Read the model definition and answer for the solid it produces. Units are mm, in the model's axes. A direction names the side the tool comes from. Coordinates: 2 decimals unless noted, no trailing zeros. Loops run counter-clockwise (first coordinate to the right, second up) from the corner with the lowest first, then second, coordinate; pieces in that order, holes last.
Autodesk Inventor part; units mm, degrees
ref_plane "YZ Plane" through (0, 0, 0) normal (1, 0, 0) x (0, 1, 0)
ref_plane "XZ Plane" through (0, 0, 0) normal (0, 1, 0) x (-1, 0, 0)
ref_plane "XY Plane" through (0, 0, 0) normal (0, 0, 1) x (1, 0, 0)
sketch "Sketch1" plane through (0, 0, 0) normal (0, 1, 0) x (-1, 0, 0)
  line L0 (-6.35, 6.35) -> (6.35, 6.35)
  line L1 (6.35, 6.35) -> (6.35, -6.35)
  line L2 (6.35, -6.35) -> (-6.35, -6.35)
  line L3 (-6.35, -6.35) -> (-6.35, 6.35)
  line L4 (-6.35, 6.35) -> (6.35, -6.35) construction
  line L5 (6.35, 6.35) -> (-6.35, -6.35) construction
  circle A0 centre (0, 0) radius 1.7
  dimension "d0" = 12.7
  dimension "d1" = 12.7
  dimension "d2" = 3.4
extrude "Extrusion1" add sketch "Sketch1" along normal blind 77.6732
ref_plane "Work Plane1" through (0, 69.9732, 0) normal (0, 1, 0) x (1, 0, 0)
sketch "Sketch2" plane through (0, 69.9732, 0) normal (0, 1, 0) x (1, 0, 0)
  circle A0 centre (0, 0) radius 1.7 construction
  circle A1 centre (0, 0) radius 3.45 construction
  line L0 (0, -3.45) -> (-2.9878, -1.725)
  line L1 (-2.9878, -1.725) -> (-2.9878, 6.35)
  line L2 (2.9878, 6.35) -> (2.9878, -1.725)
  line L3 (2.9878, -1.725) -> (0, -3.45)
  line L4 (6.35, 6.35) -> (-6.35, 6.35)
  line L5 (-2.9878, 6.35) -> (2.9878, 6.35)
  dimension "d6" = 6.9
extrude "Extrusion2" cut sketch "Sketch2" against normal blind 4.4
ref_plane "Work Plane2" through (0, 7.7, 0) normal (0, -1, 0) x (1, 0, 0)
sketch "Sketch3" plane through (0, 7.7, 0) normal (0, -1, 0) x (1, 0, 0)
  circle A0 centre (0, 0) radius 3.45 construction
  line L0 (2.9878, 1.725) -> (0, 3.45)
  line L1 (0, 3.45) -> (2.9878, 1.725)
  line L2 (2.9878, 1.725) -> (2.9878, -6.35)
  line L3 (-2.9878, -6.35) -> (-2.9878, 1.725)
  line L4 (-2.9878, 1.725) -> (0, 3.45)
  line L5 (6.35, -6.35) -> (-6.35, -6.35)
  line L6 (-2.9878, -6.35) -> (2.9878, -6.35)
  dimension "d10" = 6.9
extrude "Extrusion3" cut sketch "Sketch3" against normal blind 4.4
properties part number "standoff for walls"
Item 1: Which of the six approach directions +Z, -Z, +X, -X, +Y, -Y give full straight-line access (tool end or side, diameter ignored) to faces 5 (the face through (0, 7.7, -2)), 6 (the face through (-1, 0, 2))?
Numbers:
face 5: -Z
face 6: +Z, -Z, +X, -X, -Y
Item 2: A cutting plane is placed at B-B on y = 6. Determine the outline of the cut face in (x, z).
Numbers:
outline: (-6.35, -6.35) - (6.35, -6.35) - (6.35, 6.35) - (-6.35, 6.35) - close; hole circle Ø3.4 at (0, 0)
Item 3: Determine the mould class of faces 1 (the face through (-1.51, 9.87, 2.58)), 2 (the face through (0.37, 38.46, 1.66)), 3 (the face through (2.988, 10, -2)), 4 (the face through (-1, 77.673, 2)) for opening direction Y: released by +Y, released by -Y, zero draft, split by the parting line, or undercut.
Numbers:
face 1: undercut
face 2: zero draft
face 3: undercut
face 4: released by +Y
Item 4: A cutting plane is placed at A-A on z = 0. Determine the outline of the cut face in (x, y).
Numbers:
outline: (-6.35, 0) - (-1.7, 0) - (-1.7, 7.7) - (-2.99, 7.7) - (-2.99, 12.1) - (-1.7, 12.1) - (-1.7, 65.57) - (-2.99, 65.57) - (-2.99, 69.97) - (-1.7, 69.97) - (-1.7, 77.67) - (-6.35, 77.67) - close; (1.7, 0) - (6.35, 0) - (6.35, 77.67) - (1.7, 77.67) - (1.7, 69.97) - (2.99, 69.97) - (2.99, 65.57) - (1.7, 65.57) - (1.7, 12.1) - (2.99, 12.1) - (2.99, 7.7) - (1.7, 7.7) - close
Item 5: Find the intervals of material crossed by line 1 along X through (y, z) = (23, 0); line 2 along Z through (x, y) = (1, 33), in increasing order.
Numbers:
line 1: x = -6.35 to -1.7, 1.7 to 6.35
line 2: z = -6.35 to -1.37, 1.37 to 6.35
Item 6: Given pin 1 (2.5 mm diameter, centred on x = 0, z = 0, fed in from -Y), flat-ended and moving along its own axis, determine where the tip first touches the part or whether it passes through.
Numbers:
pin 1: passes through
